```python
from build123d import *

# Parameters (mm, degrees)
SKETCH_1_W          = 65
SKETCH_1_H          = 15
EXTRUDE_1_DEPTH     = 2
SKETCH_2_R          = 1.25
SKETCH_2_R_2        = 2.8
SKETCH_2_R_3        = 1.5
SKETCH_2_R_4        = 1
CUT_EXTRUDE_1_DEPTH = 2
SKETCH_4_R          = 1.5
EXTRUDE_2_DEPTH     = 2


with BuildPart() as part:
    # 草图1 → 凸台-拉伸1 (new body)
    with BuildSketch(Plane(origin=(0, 0, 0), x_dir=(1, 0, 0), z_dir=(0, 1, 0))):
        with Locations((-7.5, 0)):
            Rectangle(SKETCH_1_W, SKETCH_1_H)
    extrude(amount=EXTRUDE_1_DEPTH)

    # 草图2 → 切除-拉伸1 (cut)
    with BuildSketch(Plane(origin=(0, 0, 0), x_dir=(1, 0, 0), z_dir=(0, 1, 0))):
        with Locations(Location((0, 0, 0), (0, 0, 270))):
            Circle(SKETCH_2_R)
        with Locations(Location((15, 0, 0), (0, 0, 270))):
            Circle(SKETCH_2_R_2)
        with Locations(Location((-15, 0, 0), (0, 0, 90))):
            Circle(SKETCH_2_R_2)
        with Locations(Location((23, 0, 0), (0, 0, 270))):
            Circle(SKETCH_2_R)
        with Locations(Location((-23, 0, 0), (0, 0, 90))):
            Circle(SKETCH_2_R)
        with Locations(Location((-32.5, 0, 0), (0, 0, 270))):
            Circle(SKETCH_2_R_3)
        with Locations(Location((-27, 0, 0), (0, 0, 270))):
            Circle(SKETCH_2_R_4)
        with Locations(Location((-32.5, -5.5, 0), (0, 0, 270))):
            Circle(SKETCH_2_R_4)
        with Locations(Location((-38, 0, 0), (0, 0, 270))):
            Circle(SKETCH_2_R_4)
        with Locations(Location((-32.5, 5.5, 0), (0, 0, 270))):
            Circle(SKETCH_2_R_4)
    extrude(amount=CUT_EXTRUDE_1_DEPTH, mode=Mode.SUBTRACT)

    # 草图4 → 凸台-拉伸2 (add)
    with BuildSketch(Plane.XY.offset(7.5)):
        with Locations(Location((20, 1, 0), (0, 0, 221.810314896))):
            Circle(SKETCH_4_R)
        with Locations(Location((-20, 1, 0), (0, 0, 221.810314896))):
            Circle(SKETCH_4_R)
    extrude(amount=EXTRUDE_2_DEPTH)


solid = part.part
```
Can you work these out from the model? Positions are in its coordinate system, mm. A direction names the side the tool comes from. Give positions to 0.01 mm unless a question says otherwise; leave off trailing zeros. Write each loop counter-clockwise with the first axis right and the second up, starting at its lowest first coordinate (ties: lowest second). Pieces come first, ordered by that corner, then holes. Notation, with made-up numbers: (33, 48.25) - (55, 48.25) arc R20 cw to (55, 61.25) - close; hole circle Ø7 at (-1, 43.25). An arc over 180 degrees is marked (long way). Write item = value, one per line. Start each with the question number.
1. Imagine slicing it at D-D (z = -5.5). Please give me the cut outline in (x, y).
2. Imagine slicing it at C-C (y = 1). Count the separate pieces of the cut face and the enclosed holes in it, and give its area (3 significant figures).
3. Imagine slicing it at A-A (x = 23). Please give me the cut outline in (y, z), and give its area (3 significant figures).
4. Please list where these lines run through material, in increasing order: line 1 (X direction, y = 0.65, z = 5.5); line 2 (Z direction, x = 11, y = 0.3); line 3 (Y direction, x = 12.5, z = 4.25).
5. For pin 1 (2 mm diameter, centred on x = -23, z = 0, fed in from -Y); pin 2 (1 mm diameter, centred on x = 23.5, y = 0.5, fed in from +Z); pin 3 (3 mm diameter, centred on x = 0, z = 0, fed in from -Y); pin 4 (1 mm diameter, centred on x = 0.5, z = -1.5, fed in from +Y), each with a flat end and sliding along its axis, tell me the tip position at first contact or that it passes through.
6. On a 3-axis mill with a long thin cutter (end or side, diameter ignored), from which of +Z, -Z, +X, -X, +Y, -Y can I reach the whole of each face in a straight line? I mean faces 1 (the face through (-20, 1, 9.5)), 2 (the face through (-18.5, 1, 8.5)), 3 (the face through (-8, 2, 0)), 4 (the face through (-8, 0, 0)). Say none if no direction works.
7. Thinking about a two-plate mould opening in Z: for faces 5 (the face through (-28, 1, 0)), 6 (the face through (-21.78, 0.99, 0.27)), 7 (the face through (21.137, 0.022, 8.486)), 8 (the face through (0, 1, 7.5)), which applies, released by +Z, released by -Z, zero draft, split by the parting line, or undercut?
8. Imagine slicing it at B-B (x = -32.5). Please give me the cut outline in (y, z), and give its area (3 significant figures).
Worked answers:
q1.outline = (-40, 0) - (-33.5, 0) - (-33.5, 2) - (-40, 2) - close; (-31.5, 0) - (25, 0) - (25, 2) - (-31.5, 2) - close
q2.separate_pieces = 1
q2.enclosed_holes = 10
q2.area = 903 mm2
q3.outline = (0, -7.5) - (2, -7.5) - (2, -1.25) - (0, -1.25) - close; (0, 1.25) - (2, 1.25) - (2, 7.5) - (0, 7.5) - close
q3.area = 25.0 mm2
q4.line_1 = -40 to -33.5, -31.5 to 25
q4.line_2 = -7.5 to 7.5
q4.line_3 = 0 to 2
q5.pin_1 = through
q5.pin_2 = 7.5
q5.pin_3 = 0
q5.pin_4 = 2
q6.face_1 = +Z, +X, -X, +Y, -Y
q6.face_2 = +Z
q6.face_3 = -Z, +X, -X, +Y
q6.face_4 = -Z, +X, -X, -Y
q7.face_5 = undercut
q7.face_6 = undercut
q7.face_7 = zero draft
q7.face_8 = released by +Z
q8.outline = (0, -7.5) - (2, -7.5) - (2, -6.5) - (0, -6.5) - close; (0, -4.5) - (2, -4.5) - (2, -1.5) - (0, -1.5) - close; (0, 1.5) - (2, 1.5) - (2, 4.5) - (0, 4.5) - close; (0, 6.5) - (2, 6.5) - (2, 7.5) - (0, 7.5) - close
q8.area = 16.0 mm2
